The model under review builds one solid part; all positions refer to its coordinate system, in mm. Face numbers are marked on the shaded views. A direction names the side the tool comes from. Round coordinates to 2 decimals unless told otherwise and drop trailing zeros. Order: outer loops, then holes, each group sorted by start corner. A loop starts at its lowest first (then second) coordinate and runs counter-clockwise, first axis right, second up.
```python
from build123d import *

# Parameters (mm, degrees)
F3_DEPTH = 70
F4_R     = 30
F5_DEPTH = 112
F6_R     = 15
F7_DEPTH = 163


with BuildPart() as f2:
    # F1 (on Front) → F2 (revolve)
    with BuildSketch(Plane.XZ):
        Polygon((-60, -120), (-60, -250), (0, -250), (0, 0), (-70, 0), (-70, -120), align=None)
    revolve(axis=Axis((0, 0, -125), (0, 0, -1)))

    # F0 (on Front) → F3 (join, symmetric)
    with BuildSketch(Plane.XZ):
        with BuildLine():
            ThreePointArc((113.275358, 0), (147.343032, 146.027594), (242.512075, 261.904762))
            ThreePointArc((242.512075, 261.904762), (192.752359, 769.029387), (-240, 500))
            Line((-240, 500), (-125, 500))
            ThreePointArc((-125, 500), (-95.197164, 581.009259), (-20, 623.389627))
            Line((-20, 623.389627), (-20, 624.947867))
            Line((-20, 624.947867), (20, 624.947867))
            Line((20, 624.947867), (20, 623.389627))
            ThreePointArc((20, 623.389627), (97.236318, 578.549974), (124.836727, 493.613169))
            Line((124.836727, 493.613169), (0, 278.411619))
            Line((0, 278.411619), (-31.669397, 232.573897))
            ThreePointArc((-31.669397, 232.573897), (-58.197727, 223.86417), (-66.061109, 197.072774))
            Line((-66.061109, 197.072774), (-66.061109, 164.52672))
            ThreePointArc((-66.061109, 164.52672), (-98.826102, 85.146444), (-110, 0))
            Line((-110, 0), (113.275358, 0))
        make_face()
        with BuildLine():
            Line((-125, 500), (-240, 500))
            Line((-240, 500), (-240, 350))
            ThreePointArc((-240, 350), (-219.930134, 325.490945), (-191.944498, 340.333365))
            Line((-191.944498, 340.333365), (-125, 500))
        make_face()
    extrude(amount=F3_DEPTH, both=True)

    # F4 (on Front) → F5 (cut, symmetric)
    with BuildSketch(Plane.XZ):
        with Locations((0, -190)):
            Circle(F4_R)
    extrude(amount=F5_DEPTH, both=True, mode=Mode.SUBTRACT)

    # F6 (on face) → F7 (cut, symmetric)
    with BuildSketch(Plane.XZ.offset(70)):
        with Locations((-43.483209, 207.776994)):
            Circle(F6_R)
    extrude(amount=F7_DEPTH, both=True, mode=Mode.SUBTRACT)


solid = f2.part
```
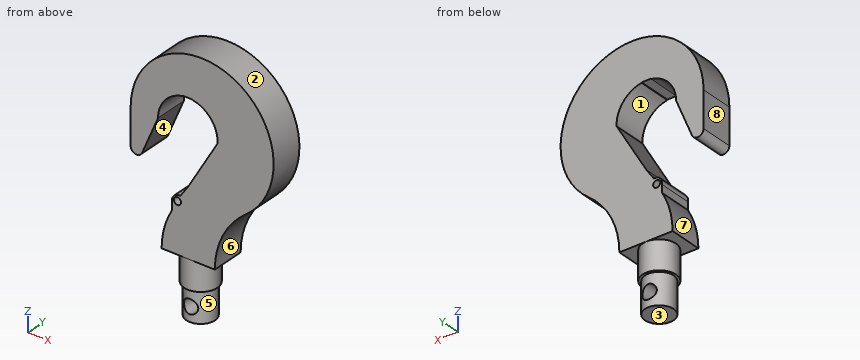
(1) Consider section C-C (z = -141). Write out the cut boundary in (x, y), and give its area (3 significant figures).
Data:
outline: circle Ø120 at (0, 0)
area: 11,300 mm2
(2) Consider section D-D (x = 226). Write out the cut boundary in (y, z).
Data:
outline: (-70, 248.38) - (70, 248.38) - (70, 749.89) - (-70, 749.89) - close
(3) Consider section A-A (x = -46.5). Write out the cut boundary in (y, z).
Data:
outline: (-70, 0) - (-52.32, 0) - (-52.32, -120) - (-37.92, -120) - (-37.92, -250) - (37.92, -250) - (37.92, -120) - (52.32, -120) - (52.32, 0) - (70, 0) - (70, 193.08) - (-70, 193.08) - close; (-70, 222.47) - (70, 222.47) - (70, 231.33) - (-70, 231.33) - close; (-70, 616.03) - (70, 616.03) - (70, 780.46) - (-70, 780.46) - close
(4) Draft analysis for pull direction Z (two halves, no side actions). For the marked faces 1, 2 and 3, state which applies: pulls with the +Z half, pulls with the -Z half, needs draft (parallel to the pull), parting line crosses it, or undercut.
Data:
face 1: undercut
face 2: parting line crosses it
face 3: pulls with the -Z half
(5) Insertion check: pin 1 (10 mm diameter, centred on x = 213.5, y = 16, fed in from -Z); pin 2 (12 mm diameter, centred on x = 179.5, y = 3.5, fed in from -Z); pin 3 (1 mm diameter, centred on y = 50.5, z = 567.5, fed in from -X). Each pin has a flat end and moves straight along its axis. Give the tip position at first contact, or say it passes through.
Data:
pin 1: stops at z = 231.91
pin 2: stops at z = 190.06
pin 3: stops at x = -232.42
(6) To check wall thickness, follow probe 1 along Y at (x, z) = (4.5, -15); probe 2 along Z at (x, y) = (0, 35); probe 3 along Z at (x, y) = (-2.5, 30.5). State the ranges of each line that lie inside material, in increasing order.
Data:
probe 1: y = -69.86 to 69.86
probe 2: z = -250 to -220, -160 to 278.41, 624.95 to 793.94
probe 3: z = -250 to -219.9, -160.1 to 274.79, 624.95 to 793.42
(7) For the marked faces 4, 5, 6, 7 and 8, list the 3-axis set-ups (+Z, -Z, +X, -X, +Y, -Y) from which the entire face can be reached by the end or side of a thin tool; tool diameter is ignored.
Data:
face 4: -Z, +Y, -Y
face 5: -Z
face 6: -Z, +X, +Y, -Y
face 7: -X, +Y, -Y
face 8: +Z, -Z, -X, +Y, -Y
(8) Consider section B-B (y = 11). Write out the cut boundary in (x, z), and give its area (3 significant figures).
Data:
outline: (-240, 350) arc R25 ccw to (-191.94, 340.33) - (-125, 500) arc R125 cw to (-20, 623.39) - (-20, 624.95) - (20, 624.95) - (20, 623.39) arc R125 cw to (124.84, 493.61) - (0, 278.41) - (-31.67, 232.57) arc R30 ccw to (-66.06, 197.07) - (-66.06, 164.53) arc R330 ccw to (-110, 0) - (-69.13, 0) - (-69.13, -120) - (-58.98, -120) - (-58.98, -250) - (58.98, -250) - (58.98, -120) - (69.13, -120) - (69.13, 0) - (113.28, 0) arc R330 cw to (242.51, 261.9) arc R300 ccw (long way) to (-240, 500) - close; hole circle Ø30 at (-43.48, 207.78); hole circle Ø60 at (0, -190)
area: 282,000 mm2
